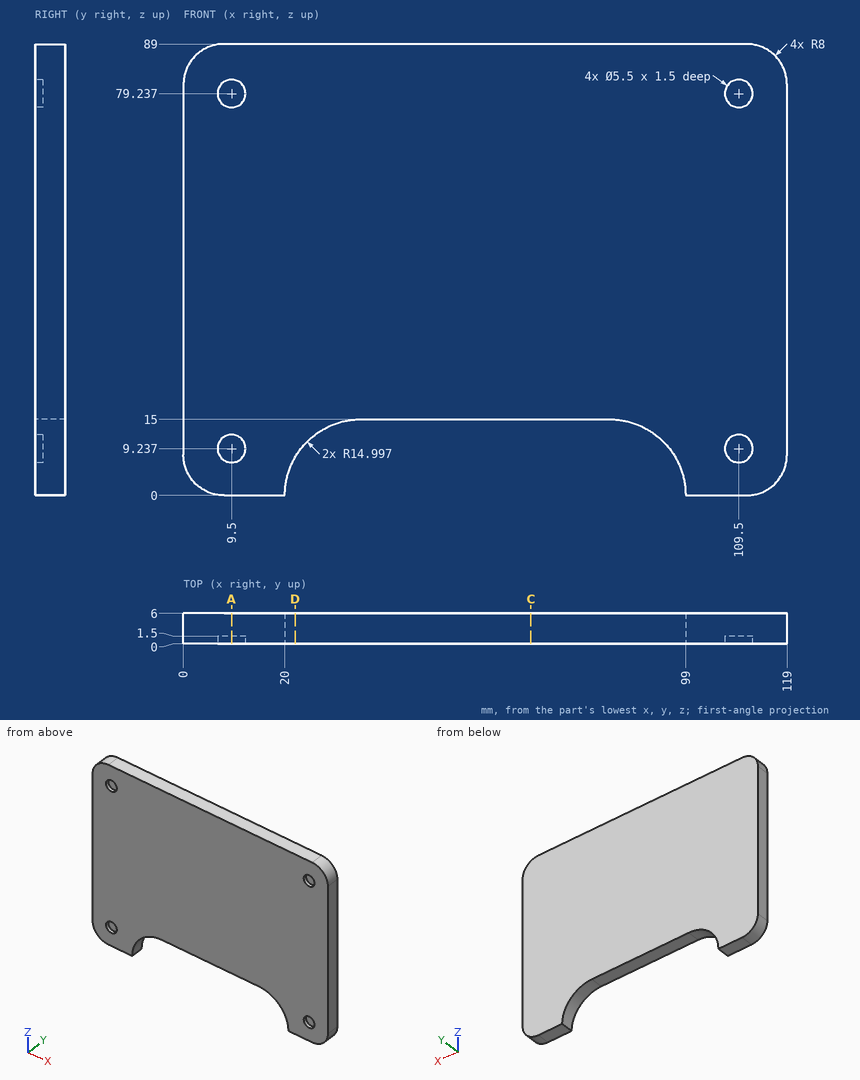
Print and shaded views of the part. All mm, measured from the part's lowest x, y and z. Give positions to 0.01 mm unless a question says otherwise; leave off trailing zeros. Write each loop counter-clockwise with the first axis right and the second up, starting at its lowest first coordinate (ties: lowest second). Pieces come first, ordered by that corner, then holes. Notation, with made-up numbers: (60, 46) - (67, 46) arc R24 ccw to (67, 78) - close; hole circle Ø5 at (35, 13). An arc over 180 degrees is marked (long way). One line per question, with ' | ' between items. Start each with the question number.
(1) Slice it at C-C on x = 68.5. Write the cut outline in (y, z), plus the area to 3 significant figures.
(2) Slice it at D-D on x = 22. Write the cut outline in (y, z).
(3) Slice it at A-A on x = 9.5. Write the cut outline in (y, z).
(4) Pin check, flat tips, straight feed: P1, Ø1.6, axis at x = 110.5, z = 80, coming from the -Y side; P2, Ø3, axis at x = 68, y = 3.5, coming from the -Z side. Stop position of each tip, or through.
(5) Wall check: line 1 along Z through (x, y) = (9.5, 0.7); line 2 along Z through (x, y) = (71, 1.6); line 3 along X through (y, z) = (5.1, 13). Give the ranges that are in metal, low to high. Write a range as from..to.
Results below:
1) outline: (0, 15) - (6, 15) - (6, 89) - (0, 89) - close | area: 444 mm^2
2) outline: (0, 7.49) - (6, 7.49) - (6, 89) - (0, 89) - close
3) outline: (0, 0) - (6, 0) - (6, 89) - (0, 89) - (0, 81.99) - (1.5, 81.99) - (1.5, 76.49) - (0, 76.49) - (0, 11.99) - (1.5, 11.99) - (1.5, 6.49) - (0, 6.49) - close
4) P1: y = 1.5 | P2: z = 15
5) line 1: 0..6.49, 11.99..76.49, 81.99..89 | line 2: 15..89 | line 3: 0..27.51, 91.49..119
